Geometry: final body of the model. Coordinates: model frame, mm. A direction names the side the tool comes from. Coordinates: 2 decimals unless noted, no trailing zeros. Loops run counter-clockwise (first coordinate to the right, second up) from the corner with the lowest first, then second, coordinate; pieces in that order, holes last. Notation, with made-up numbers: (18, 7) - (49, 7) arc R23 ccw to (49, 28) - close; hole circle Ø6 at (8, 87.25). An arc over 180 degrees is marked (long way). Put each result on its own line as item: value. Start each with the question number.
1) Contact query for a flat-ended pin moving along its axis: pin 1 Ø12 at (x, y) = (574, -219) entering from +Z. Output: stop coordinate, or through.
2) Section C-C on x = 150. Output: boundary loops of the cut face in (y, z).
3) Section B-B on y = -343. Output: boundary loops of the cut face in (x, z), and give its area (3 significant figures).
4) Draft query along X for faces 3 (the flat face through (444, -276, 0)), 4 (the flat face through (0, -276, 355)), 5 (the flat face through (444, -285, 18)), 6 (the flat face through (900, -276, 355)). Return one class per face: +X half, -X half, draft (parallel to the pull), parting line (faces both ways), or undercut.
5) Section A-A on z = 172. Output: boundary loops of the cut face in (x, y).
6) Reachability of faces 1 (the flat face through (248, -9, 720)), 2 (the flat face through (18, -285, 364)) from +Z, -Z, +X, -X, +Y, -Y: full face, straight path, thin tool, end or side. Return the list, or none.
7) Material intervals for line 1 along X through (y, z) = (-44, 194); line 2 along Z through (x, y) = (158, -453.5); line 3 along Y through (x, z) = (689, 48), sorted ascending. Write a range as from..to.
```python
from build123d import *

# Parameters (mm, degrees)
F0_W     = 51.5153110027
F0_H     = 46.9279363751
F1_DEPTH = 560
F2_DEPTH = 900
F3_DEPTH = 720
F4_T     = -18


with BuildPart() as f1:
    # F0 (on Front) → F1 (new body)
    with BuildSketch(Plane.XZ):
        with Locations((25.7576555014, 23.4639681876)):
            Rectangle(F0_W, F0_H)
    extrude(amount=F1_DEPTH)

    # F2 (add): a face of the model
    f2_faces = [f1.faces().sort_by_distance(p)[0] for p in [
        (0, -280, 23.4639681876),
    ]]
    extrude(f2_faces, amount=-F2_DEPTH)

    # F3 (add): a face of the model
    f3_faces = [f1.faces().sort_by_distance(p)[0] for p in [
        (450, -280, 0),
    ]]
    extrude(f3_faces, amount=-F3_DEPTH)

    # F4
    f4_openings = [f1.faces().sort_by_distance(p)[0] for p in [
        (450, -560, 360),
        (450, -280, 720),
    ]]
    offset(amount=F4_T, openings=f4_openings)


solid = f1.part
```
Answer block:
1. pin 1: stops at z = 18
2. outline: (-560, 0) - (0, 0) - (0, 720) - (-18, 720) - (-18, 18) - (-560, 18) - close
3. outline: (0, 0) - (900, 0) - (900, 720) - (882, 720) - (882, 18) - (18, 18) - (18, 720) - (0, 720) - close
3. area: 41,500 mm²
4. face 3: draft
4. face 4: -X half
4. face 5: undercut
4. face 6: +X half
5. outline: (0, -560) - (18, -560) - (18, -18) - (882, -18) - (882, -560) - (900, -560) - (900, 0) - (0, 0) - close
6. face 1: +Z, +X, -X, +Y, -Y
6. face 2: +Z, -Y
7. line 1: x = 0..18, 882..900
7. line 2: z = 0..18
7. line 3: y = -18..0
